from build123d import *

# Parameters (mm, degrees)
SKETCH1_W           = 361.95
SKETCH1_H           = 215.9
BOSS_EXTRUDE1_DEPTH = 10
FILLET1_R           = 5
BOSS_EXTRUDE2_START = 15
BOSS_EXTRUDE2_DEPTH = 15
FILLET2_R           = 5
SKETCH3_R           = 38.02
BOSS_EXTRUDE3_DEPTH = 30
SKETCH4_R           = 34.02
CUT_EXTRUDE1_DEPTH  = 25
CHAMFER1_SIZE       = 15
CHAMFER2_SIZE       = 5
FILLET3_R           = 2.5
SKETCH6_W           = 150
SKETCH6_H           = 75
BOSS_EXTRUDE4_DEPTH = 20
SKETCH5_W           = 140
SKETCH5_H           = 65
CUT_EXTRUDE2_DEPTH  = 25
FILLET4_R           = 2.5
FILLET5_R           = 2.5


with BuildPart() as part:
    # Sketch1 → Boss-Extrude1 (new body)
    with BuildSketch(Plane(origin=(0, 0, 0), x_dir=(1, 0, 0), z_dir=(0, 1, 0))):
        Rectangle(SKETCH1_W, SKETCH1_H)
    extrude(amount=BOSS_EXTRUDE1_DEPTH)

    # Fillet1
    fillet1_edges = [part.edges().sort_by_distance(p)[0] for p in [
        (-180.975, 5, 107.95),
        (-180.975, 5, -107.95),
        (180.975, 5, -107.95),
        (180.975, 5, 107.95),
    ]]
    fillet(fillet1_edges, radius=FILLET1_R)

    # Sketch2 → Boss-Extrude2 (add)
    with BuildSketch(Plane(origin=(0, 10, 0), x_dir=(1, 0, 0), z_dir=(0, 1, 0)).offset(BOSS_EXTRUDE2_START)):
        with BuildLine():
            Line((-175.975, -107.95), (175.975, -107.95))
            ThreePointArc((175.975, -107.95), (179.510533906, -106.485533906), (180.975, -102.95))
            Line((180.975, -102.95), (180.975, 102.95))
            ThreePointArc((180.975, 102.95), (179.510533906, 106.485533906), (175.975, 107.95))
            Line((175.975, 107.95), (-175.975, 107.95))
            ThreePointArc((-175.975, 107.95), (-179.510533906, 106.485533906), (-180.975, 102.95))
            Line((-180.975, 102.95), (-180.975, -102.95))
            ThreePointArc((-180.975, -102.95), (-179.510533906, -106.485533906), (-175.975, -107.95))
        make_face()
        with BuildLine():
            Line((-165.975, -97.95), (165.975, -97.95))
            ThreePointArc((165.975, -97.95), (169.510533906, -96.485533906), (170.975, -92.95))
            Line((170.975, -92.95), (170.975, 92.95))
            ThreePointArc((170.975, 92.95), (169.510533906, 96.485533906), (165.975, 97.95))
            Line((165.975, 97.95), (-165.975, 97.95))
            ThreePointArc((-165.975, 97.95), (-169.510533906, 96.485533906), (-170.975, 92.95))
            Line((-170.975, 92.95), (-170.975, -92.95))
            ThreePointArc((-170.975, -92.95), (-169.510533906, -96.485533906), (-165.975, -97.95))
        make_face(mode=Mode.SUBTRACT)
    extrude(amount=-BOSS_EXTRUDE2_DEPTH)

    # Fillet2
    fillet2_edges = [part.edges().sort_by_distance(p)[0] for p in [
        (0, 10, 97.95),
        (169.510533906, 10, 96.485533906),
        (170.975, 10, 0),
        (169.510533906, 10, -96.485533906),
        (0, 10, -97.95),
        (-169.510533906, 10, -96.485533906),
        (-170.975, 10, 0),
        (-169.510533906, 10, 96.485533906),
    ]]
    fillet(fillet2_edges, radius=FILLET2_R)

    # Sketch3 → Boss-Extrude3 (add)
    with BuildSketch(Plane(origin=(0, 10, 0), x_dir=(1, 0, 0), z_dir=(0, 1, 0))):
        with Locations(Location((-90.4875, 46.475, 0), (0, 0, 270))):
            Circle(SKETCH3_R)
    extrude(amount=-BOSS_EXTRUDE3_DEPTH)

    # Sketch4 → Cut-Extrude1 (cut)
    with BuildSketch(Plane(origin=(0, 10, 0), x_dir=(1, 0, 0), z_dir=(0, 1, 0))):
        with Locations(Location((-90.4875, 46.475, 0), (0, 0, 270))):
            Circle(SKETCH4_R)
    extrude(amount=-CUT_EXTRUDE1_DEPTH, mode=Mode.SUBTRACT)

    # Chamfer1
    chamfer1_edges = [part.edges().sort_by_distance(p)[0] for p in [
        (-90.4875, 0, -84.495),
    ]]
    chamfer(chamfer1_edges, length=CHAMFER1_SIZE)

    # Chamfer2
    chamfer2_edges = [part.edges().sort_by_distance(p)[0] for p in [
        (-90.4875, 10, -80.495),
    ]]
    chamfer(chamfer2_edges, length=CHAMFER2_SIZE)

    # Fillet3
    fillet3_edges = [part.edges().sort_by_distance(p)[0] for p in [
        (-90.4875, -15, -80.495),
    ]]
    fillet(fillet3_edges, radius=FILLET3_R)

    # Sketch6 → Boss-Extrude4 (add)
    with BuildSketch(Plane.XZ):
        with Locations((-54.5075, 46.475)):
            Rectangle(SKETCH6_W, SKETCH6_H)
    extrude(amount=BOSS_EXTRUDE4_DEPTH)

    # Sketch5 → Cut-Extrude2 (cut)
    with BuildSketch(Plane(origin=(0, 10, 0), x_dir=(1, 0, 0), z_dir=(0, 1, 0))):
        with Locations((-54.5075, -46.475)):
            Rectangle(SKETCH5_W, SKETCH5_H)
    extrude(amount=-CUT_EXTRUDE2_DEPTH, mode=Mode.SUBTRACT)

    # Fillet4
    fillet4_edges = [part.edges().sort_by_distance(p)[0] for p in [
        (-129.5075, -20, 46.475),
        (-129.5075, -10, 83.975),
        (-54.5075, 0, 8.975),
        (-129.5075, -10, 8.975),
        (20.4925, 0, 46.475),
        (20.4925, -10, 8.975),
        (-54.5075, -20, 83.975),
        (20.4925, -10, 83.975),
        (-54.5075, -20, 8.975),
        (20.4925, -20, 46.475),
        (-129.5075, 0, 46.475),
        (-54.5075, 0, 83.975),
    ]]
    fillet(fillet4_edges, radius=FILLET4_R)

    # Fillet5
    fillet5_edges = [part.edges().sort_by_distance(p)[0] for p in [
        (-54.5075, 10, 13.975),
        (-124.5075, -2.5, 13.975),
        (15.4925, 10, 46.475),
        (15.4925, -2.5, 13.975),
        (-54.5075, -15, 78.975),
        (15.4925, -2.5, 78.975),
        (-124.5075, -15, 46.475),
        (-124.5075, -2.5, 78.975),
        (-54.5075, -15, 13.975),
        (15.4925, -15, 46.475),
        (-124.5075, 10, 46.475),
        (-54.5075, 10, 78.975),
    ]]
    fillet(fillet5_edges, radius=FILLET5_R)


solid = part.part
Source: CAD feature listing. Evaluate the final solid. Frame: model axes, mm. A direction names the side the tool comes from. Round coordinates to 2 decimals unless told otherwise and drop trailing zeros. Write each loop counter-clockwise with the first axis right and the second up, starting at its lowest first coordinate (ties: lowest second). Pieces come first, ordered by that corner, then holes. Notation, with made-up numbers: (12.5, -2) - (54.5, -2) arc R22 cw to (54.5, 20) - close; hole circle Ø3 at (87.25, -34). An arc over 180 degrees is marked (long way). Use CSV: the item, a comma, the result in double quotes. Start each with the question number.
(1) First-contact query: pin 1 Ø16.5 at (x, y) = (-49, -9) entering from -Z; pin 2 Ø1 at (y, z) = (-12.5, 58) entering from -X; pin 3 Ø1 at (x, z) = (143, 50.5) entering from +Y. Flat tips, straight axial feed; report the tip coordinate or a pass-through.
(2) Cut plane C-C, the plane z = 46.5. Return loops of the section in (x, y) (1 decimal).
(3) Cut plane A-A, the plane y = 19.5. Return loops of the section in (x, z) (3 decimals).
(4) Set-up query: faces 4 (the face through (-170.975, 20, -1)), 5 (the face through (20.492, -10, 46)), 6 (the face through (-58.429, -17.465, -26.036)), 7 (the face through (-56, -10, 8.975)). Return all of +Z, -Z, +X, -X, +Y, -Y with unobstructed straight access to the full face (end or side cutting, diameter ignored); none if empty.
(5) Mould query, pull axis Z, two halves, no side actions, for faces 1 (the face through (39, 10, -1)), 2 (the face through (-56, -10, 83.975)), 3 (the face through (-56, -20, 47)). Classes: pulls with the +Z half, pulls with the -Z half, needs draft (parallel to the pull), parting line crosses it, or undercut.
(6) Cut plane B-B, the plane x = 158. Return loops of the section in (y, z).
(7) Material intervals for probe 1 along Z at (x, y) = (-82, -9.5) (3 decimals); probe 2 along Z at (x, y) = (7, -5.5) (3 decimals); probe 3 along Z at (x, y) = (-29, 15), sorted ascending. Write a range as [from, to].
Geometry says:
1,pin 1,"z = -81.51"
1,pin 2,"x = -129.51"
1,pin 3,"y = 10"
2,outline,"(-181, 0) - (-132, 0) arc R2.5 cw to (-129.5, -2.5) - (-129.5, -17.5) arc R2.5 ccw to (-127, -20) - (18, -20) arc R2.5 ccw to (20.5, -17.5) - (20.5, -2.5) arc R2.5 cw to (23, 0) - (181, 0) - (181, 25) - (171, 25) - (171, 15) arc R5 cw to (166, 10) - (18, 10) arc R2.5 ccw to (15.5, 7.5) - (15.5, -12.5) arc R2.5 cw to (13, -15) - (-122, -15) arc R2.5 cw to (-124.5, -12.5) - (-124.5, 7.5) arc R2.5 ccw to (-127, 10) - (-166, 10) arc R5 cw to (-171, 15) - (-171, 25) - (-181, 25) - close"
3,outline,"(-180.975, -102.95) arc R5 ccw to (-175.975, -107.95) - (175.975, -107.95) arc R5 ccw to (180.975, -102.95) - (180.975, 102.95) arc R5 ccw to (175.975, 107.95) - (-175.975, 107.95) arc R5 ccw to (-180.975, 102.95) - close; hole (-170.975, -92.95) arc R5 ccw to (-165.975, -97.95) - (165.975, -97.95) arc R5 ccw to (170.975, -92.95) - (170.975, 92.95) arc R5 ccw to (165.975, 97.95) - (-165.975, 97.95) arc R5 ccw to (-170.975, 92.95) - close"
4,face 4,"+Y"
4,face 5,"+Z, -Z, +X, -Y"
4,face 6,"-Y"
4,face 7,"+X, -X, -Y"
5,face 1,"undercut"
5,face 2,"pulls with the +Z half"
5,face 3,"needs draft"
6,outline,"(0, -107.95) - (25, -107.95) - (25, -97.95) - (15, -97.95) arc R5 cw to (10, -92.95) - (10, 92.95) arc R5 cw to (15, 97.95) - (25, 97.95) - (25, 107.95) - (0, 107.95) - close"
7,probe 1,"[-89.159, -79.419], [-13.531, -3.791], [8.975, 13.975], [78.975, 83.975]"
7,probe 2,"[8.975, 13.975], [78.975, 83.975]"
7,probe 3,"[-107.95, -97.95], [97.95, 107.95]"
